Source: CAD feature listing. Evaluate the final solid. Frame: model axes, mm. A direction names the side the tool comes from. Round coordinates to 2 decimals unless told otherwise and drop trailing zeros. Write each loop counter-clockwise with the first axis right and the second up, starting at its lowest first coordinate (ties: lowest second). Pieces come first, ordered by that corner, then holes.
from build123d import *

# Parameters (mm, degrees)
BOSS_EXTRUDE1_DEPTH       = 6.35
SKETCH2_W                 = 12.7
SKETCH2_H                 = 12.7
BOSS_EXTRUDE2_DEPTH       = 12.7
CUT_EXTRUDE1_DEPTH        = 4.445
CUT_EXTRUDE1_DEPTH_BACK   = 4.445
CUT_EXTRUDE1_START        = 6.35
SKETCH3_W                 = 8.89
SKETCH3_H                 = 8.89
F_8_32_TAPPED_HOLE1_D     = 3.4544
F_8_32_TAPPED_HOLE1_DEPTH = 12.28344
F_8_32_TAPPED_HOLE1_TIP   = 1.037806461
F_8_32_TAPPED_HOLE2_D     = 3.4544
F_8_32_TAPPED_HOLE2_DEPTH = 12.192
F_8_32_TAPPED_HOLE2_TIP   = 1.037806461
F_8_32_TAPPED_HOLE3_D     = 3.4544
F_8_32_TAPPED_HOLE3_DEPTH = 12.192
F_8_32_TAPPED_HOLE3_TIP   = 1.037806461
F_8_32_TAPPED_HOLE4_D     = 3.4544
F_8_32_TAPPED_HOLE4_DEPTH = 12.192
F_8_32_TAPPED_HOLE4_TIP   = 1.037806461


with BuildPart() as part:
    # Sketch1 → Boss-Extrude1 (new body)
    with BuildSketch(Plane(origin=(0, 0, 0), x_dir=(1, 0, 0), z_dir=(0, 1, 0))):
        Polygon((0, 0), (19.05, 3.359028982), (19.05, 9.340971018), (0, 12.7), align=None)
    extrude(amount=BOSS_EXTRUDE1_DEPTH)

    # Sketch2 → Boss-Extrude2 (add)
    with BuildSketch(Plane(origin=(0, 0, 0), x_dir=(1, 0, 0), z_dir=(0, 1, 0))):
        with Locations((-6.35, 6.35)):
            Rectangle(SKETCH2_W, SKETCH2_H)
    extrude(amount=BOSS_EXTRUDE2_DEPTH)

    # Sketch3 → Cut-Extrude1 (cut, two sides: drawn at the far end of the back side and taken through both)
    with BuildSketch(Plane(origin=(0, 0, 0), x_dir=(1, 0, 0), z_dir=(0, 1, 0)).offset(CUT_EXTRUDE1_START - CUT_EXTRUDE1_DEPTH_BACK)):
        with Locations((-6.35, 6.421317362)):
            Rectangle(SKETCH3_W, SKETCH3_H)
    extrude(amount=CUT_EXTRUDE1_DEPTH + CUT_EXTRUDE1_DEPTH_BACK, mode=Mode.SUBTRACT)

    # #8-32 Tapped Hole1
    with Locations(Plane.XY):
        with Locations((-6.210106544, 6.467962425), (-17.791429467, 4.563139576)):
            Hole(F_8_32_TAPPED_HOLE1_D / 2, depth=F_8_32_TAPPED_HOLE1_DEPTH)
            with Locations((0, 0, -(F_8_32_TAPPED_HOLE1_DEPTH + F_8_32_TAPPED_HOLE1_TIP / 2))):  # 118° drill point
                Cone(0, F_8_32_TAPPED_HOLE1_D / 2, F_8_32_TAPPED_HOLE1_TIP, mode=Mode.SUBTRACT)

    # #8-32 Tapped Hole2
    with Locations(Plane(origin=(0, 0, -12.7), x_dir=(-1, 0, 0), z_dir=(0, 0, -1))):
        with Locations((6.210106544, 6.467962425)):
            Hole(F_8_32_TAPPED_HOLE2_D / 2, depth=F_8_32_TAPPED_HOLE2_DEPTH)
            with Locations((0, 0, -(F_8_32_TAPPED_HOLE2_DEPTH + F_8_32_TAPPED_HOLE2_TIP / 2))):  # 118° drill point
                Cone(0, F_8_32_TAPPED_HOLE2_D / 2, F_8_32_TAPPED_HOLE2_TIP, mode=Mode.SUBTRACT)

    # #8-32 Tapped Hole3
    with Locations(Plane(origin=(0, 12.7, 0), x_dir=(1, 0, 0), z_dir=(0, 1, 0))):
        with Locations((-6.284915842, 6.460616317)):
            Hole(F_8_32_TAPPED_HOLE3_D / 2, depth=F_8_32_TAPPED_HOLE3_DEPTH)
            with Locations((0, 0, -(F_8_32_TAPPED_HOLE3_DEPTH + F_8_32_TAPPED_HOLE3_TIP / 2))):  # 118° drill point
                Cone(0, F_8_32_TAPPED_HOLE3_D / 2, F_8_32_TAPPED_HOLE3_TIP, mode=Mode.SUBTRACT)

    # #8-32 Tapped Hole4
    with Locations(Plane.ZY.offset(12.7)):
        with Locations((-6.409821041, 6.541174093)):
            Hole(F_8_32_TAPPED_HOLE4_D / 2, depth=F_8_32_TAPPED_HOLE4_DEPTH)
            with Locations((0, 0, -(F_8_32_TAPPED_HOLE4_DEPTH + F_8_32_TAPPED_HOLE4_TIP / 2))):  # 118° drill point
                Cone(0, F_8_32_TAPPED_HOLE4_D / 2, F_8_32_TAPPED_HOLE4_TIP, mode=Mode.SUBTRACT)


solid = part.part
1) Reachability of faces 5 (the face through (-11.734, 7.06, -8.057)), 6 (the face through (0, 9, -6)), 7 (the face through (-1.905, 4, -6)) from +Z, -Z, +X, -X, +Y, -Y: full face, straight path, thin tool, end or side. Return the list, or none.
Taken from the geometry:
face 5: -X
face 6: +Z, -Z, +X, +Y
face 7: none
2) Pull-direction query (X, two-part tool) for faces 1 (the face through (-12.7, 5, -5)), 2 (the face through (9.392, 3.131, -1.656)), 3 (the face through (-8.4, 6.3, -1.976)), 4 (the face through (-10.795, 4, -6)); classes: released by +X, released by -X, zero draft, split by the parting line, or undercut.
Taken from the geometry:
face 1: released by -X
face 2: released by +X
face 3: undercut
face 4: undercut
3) Material intervals for line 1 (X direction, y = 6.5, z = -3.75) (3 decimals); line 2 (Y direction, x = -10, z = -9.5) (3 decimals); line 3 (X direction, y = 3.5, z = -5.25) (3 decimals), sorted ascending.
Taken from the geometry:
line 1: x = -12.7 to -10.795, -1.905 to 0
line 2: y = 0 to 1.905, 10.795 to 12.7
line 3: x = -12.7 to -10.795, -1.905 to 19.05
4) Section query A-A on y = 4.25. Return the cut outline in (x, z) (3 decimals).
Taken from the geometry:
outline: (-12.7, -12.7) - (0, -12.7) - (19.05, -9.341) - (19.05, -3.359) - (0, 0) - (-12.7, 0) - close; hole (-10.795, -10.866) - (-1.905, -10.866) - (-1.905, -1.976) - (-10.795, -1.976) - close
5) Section query C-C on z = -1.25. Return the cut outline in (x, y).
Taken from the geometry:
outline: (-12.7, 0) - (7.09, 0) - (7.09, 6.35) - (0, 6.35) - (0, 12.7) - (-12.7, 12.7) - close; hole circle Ø3.45 at (-6.21, 6.47)
6) Section query D-D on y = 8.75. Return the cut outline in (x, z) (3 decimals).
Taken from the geometry:
outline: (-12.7, -12.7) - (0, -12.7) - (0, 0) - (-12.7, 0) - close; hole (-10.795, -10.866) - (-1.905, -10.866) - (-1.905, -1.976) - (-10.795, -1.976) - close
7) Section query B-B on x = -9. Return the cut outline in (y, z) (3 decimals).
Taken from the geometry:
outline: (0, -12.7) - (12.7, -12.7) - (12.7, 0) - (0, 0) - close; hole (1.905, -10.866) - (10.795, -10.866) - (10.795, -1.976) - (1.905, -1.976) - close
8) Contact query for flat-ended pins moving along their axis: P1, Ø2, axis at x = 8, y = 4, coming from the +Z side; P2, Ø6, axis at x = 11.5, z = -4, coming from the +Y side. Output: stop coordinate, or through.
Taken from the geometry:
P1: stops at z = -1.23
P2: stops at y = 6.35
